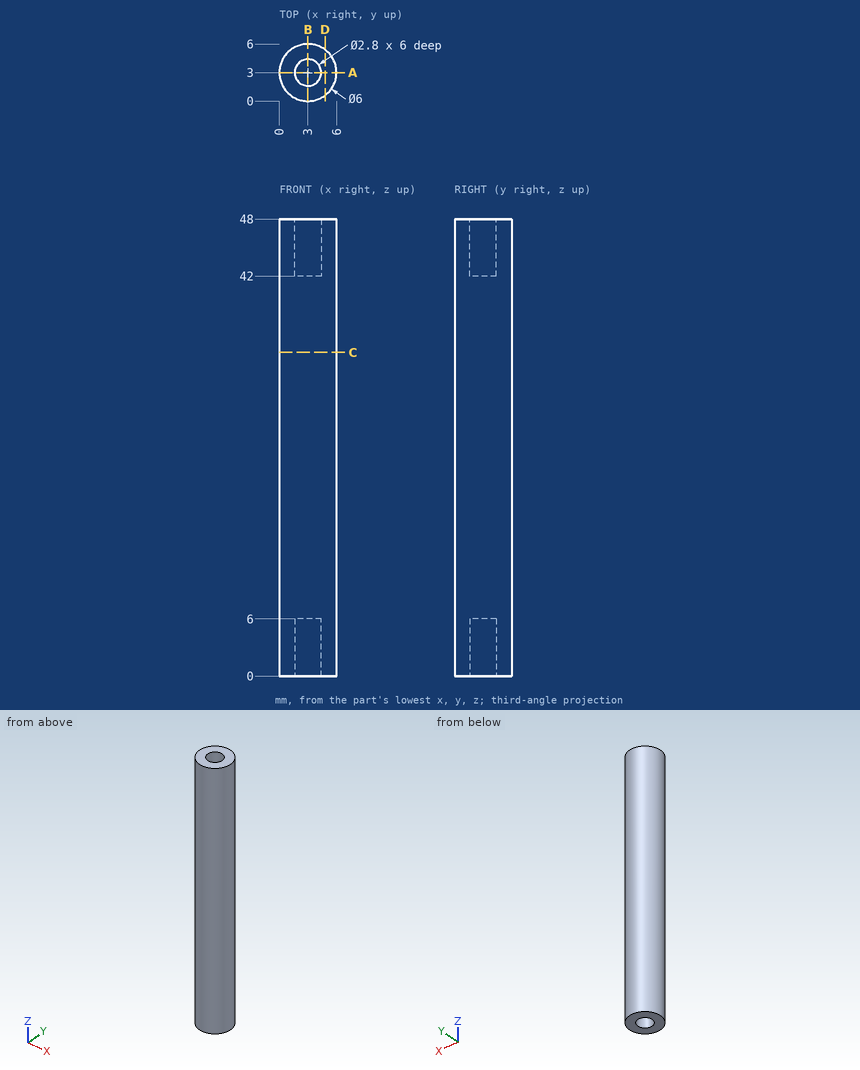
Can you work these out from the drawing? Everything is in mm from the part's minimum corner. Round coordinates to 2 decimals unless told otherwise and drop trailing zeros. Order: outer loops, then holes, each group sorted by start corner. A loop starts at its lowest first (then second) coordinate and runs counter-clockwise, first axis right, second up. Notation, with made-up numbers: (21, 9.25) -> (70, 9.25) arc R31 ccw to (70, 45.25) -> close; hole circle Ø3 at (21.5, 68.5). An arc over 180 degrees is marked (long way). Return JSON: item names as keys, results as strings. Group by question number.
1. If we section it at A-A, the plane y = 3: Write out the boundary of the cut face in (x, z), then the cut area to 3 significant figures.
2. If we section it at C-C, the plane z = 34: Write out the boundary of the cut face in (x, y), then the cut area to 3 significant figures.
3. Will these pins go through, and if not, where does the flat tip stop? pin 1 (1.7 mm diameter, centred on x = 3, y = 3, fed in from +Z); pin 2 (1 mm diameter, centred on x = 4.5, z = 18, fed in from +Y); pin 3 (1 mm diameter, centred on y = 0.5, z = 26, fed in from -X).
4. I need wall thicknesses on line 1 (Y direction, x = 3, z = 1.4); line 2 (Y direction, x = 2.8, z = 31.5); line 3 (Y direction, x = 0.35, z = 24.5). Which ranges of each line are inside material? Lowest first, please. Write a range as [from, to].
5. If we section it at D-D, the plane x = 4.8: Write out the boundary of the cut face in (y, z), then the cut area to 3 significant figures.
Output values:
{
 "1": {"outline": "(0, 0) -> (1.6, 0) -> (1.6, 6) -> (4.4, 6) -> (4.4, 0) -> (6, 0) -> (6, 48) -> (4.4, 48) -> (4.4, 42) -> (1.6, 42) -> (1.6, 48) -> (0, 48) -> close", "area": "254 mm²"},
 "2": {"outline": "circle Ø6 at (3, 3)", "area": "28.3 mm²"},
 "3": {"pin 1": "z = 42", "pin 2": "y = 5.83", "pin 3": "x = 0.76"},
 "4": {"line 1": "[0, 1.6], [4.4, 6]", "line 2": "[0.01, 5.99]", "line 3": "[1.59, 4.41]"},
 "5": {"outline": "(0.6, 0) -> (5.4, 0) -> (5.4, 48) -> (0.6, 48) -> close", "area": "230 mm²"}
}
